Can you work these out from the model? Positions are in its coordinate system, mm. A direction names the side the tool comes from. Round coordinates to 2 decimals unless told otherwise and drop trailing zeros. Order: outer loops, then holes, each group sorted by start corner. A loop starts at its lowest first (then second) coordinate and runs counter-clockwise, first axis right, second up. Notation, with made-up numbers: (-27.5, -16.75) - (-0.5, -16.75) arc R20 ccw to (-0.5, 18.25) - close; hole circle Ø7 at (63.25, 22.25). An arc over 180 degrees is marked (long way). Write item = value, one per line.
Autodesk Fusion 360 part; units mm, degrees
sketch "Sketch1" plane through (0, 0, 0) normal (0, 1, 0) x (1, 0, 0)
  line L0 (0, 0) -> (89, 0)
  line L1 (89, 0) -> (89, -113)
  line L2 (89, -113) -> (0, -113)
  line L3 (0, -113) -> (0, 0)
  line L4 (0, 0) -> (4, 0)
  line L5 (4, 0) -> (4, -4)
  line L6 (4, -4) -> (0, -4)
  line L7 (0, -4) -> (0, 0)
  line L8 (89, 0) -> (85, 0)
  line L9 (85, 0) -> (85, -4)
  line L10 (85, -4) -> (89, -4)
  line L11 (89, -4) -> (89, 0)
  line L12 (89, -113) -> (85, -113)
  line L13 (85, -113) -> (85, -109)
  line L14 (85, -109) -> (89, -109)
  line L15 (89, -109) -> (89, -113)
  line L16 (0, -113) -> (4, -113)
  line L17 (4, -113) -> (4, -109)
  line L18 (4, -109) -> (0, -109)
  line L19 (0, -109) -> (0, -113)
  circle A0 centre (4, -4) radius 1.1
  circle A1 centre (85, -4) radius 1.1
  circle A2 centre (85, -109) radius 1.1
  circle A3 centre (4, -109) radius 1.1
  circle A4 centre (20, -20) radius 2.5
  line L20 (89, 0) -> (69, 0)
  line L21 (69, 0) -> (69, -20)
  line L22 (69, -20) -> (89, -20)
  line L23 (89, -20) -> (89, 0)
  line L24 (0, 0) -> (20, 0)
  line L25 (20, 0) -> (20, -20)
  line L26 (20, -20) -> (0, -20)
  line L27 (0, -20) -> (0, 0)
  line L28 (0, -113) -> (20, -113)
  line L29 (20, -113) -> (20, -93)
  line L30 (20, -93) -> (0, -93)
  line L31 (0, -93) -> (0, -113)
  line L32 (89, -113) -> (69, -113)
  line L33 (69, -113) -> (69, -93)
  line L34 (69, -93) -> (89, -93)
  line L35 (89, -93) -> (89, -113)
  circle A5 centre (69, -20) radius 2.5
  circle A6 centre (20, -93) radius 2.5
  circle A7 centre (69, -93) radius 2.5
  dimension "d1" = 89
  dimension "d2" = 113
  dimension "d3" = 4
  dimension "d4" = 4
  dimension "d5" = 4
  dimension "d6" = 4
  dimension "d7" = 4
  dimension "d8" = 4
  dimension "d9" = 4
  dimension "d10" = 4
  dimension "d11" = 2.2
  dimension "d12" = 2.2
  dimension "d13" = 2.2
  dimension "d14" = 2.2
  dimension "d30" = 5
  dimension "d31" = 20
  dimension "d32" = 20
  dimension "d33" = 20
  dimension "d34" = 20
  dimension "d35" = 20
  dimension "d36" = 20
  dimension "d37" = 5
  dimension "d38" = 5
  dimension "d39" = 5
extrude "Extrude1" add sketch "Sketch1" along normal blind 2
sketch "Sketch2" plane through (0, 2, 0) normal (0, 1, 0) x (-1, 0, 0)
  line L0 (0, 0) -> (0, 113)
  line L1 (0, 113) -> (-89, 113)
  line L2 (-89, 113) -> (-89, 0)
  line L3 (-89, 0) -> (0, 0)
  line L4 (0, 0) -> (-89, 0)
  line L5 (-89, 0) -> (-89, 3.5)
  line L6 (-89, 3.5) -> (0, 3.5)
  line L7 (0, 3.5) -> (0, 0)
  line L8 (0, 0) -> (-3.5, 0)
  line L9 (-3.5, 0) -> (-3.5, 113)
  line L10 (-3.5, 113) -> (0, 113)
  line L11 (0, 113) -> (0, 0)
  line L12 (0, 113) -> (-89, 113)
  line L13 (-89, 113) -> (-89, 109.5)
  line L14 (-89, 109.5) -> (0, 109.5)
  line L15 (0, 109.5) -> (0, 113)
  line L16 (-89, 113) -> (-85.5, 113)
  line L17 (-85.5, 113) -> (-85.5, 0)
  line L18 (-85.5, 0) -> (-89, 0)
  line L19 (-89, 0) -> (-89, 113)
  dimension "d17" = 3.5
  dimension "d18" = 3.5
  dimension "d19" = 3.5
  dimension "d20" = 3.5
extrude "Extrude2" add sketch "Sketch2" along normal blind 33 contours L0 L3 L4 L6 L7 L8 L9 L11 | L0 L6 L9 L11 L14 | L3 L4 L6 L9 L17 | L0 L1 L9 L10 L11 L12 L14 L15 | L2 L3 L4 L5 L6 L17 L18 L19 | L1 L9 L12 L14 L17 | L2 L6 L14 L17 L19 | L1 L2 L12 L13 L14 L16 L17 L19
sketch "Sketch3" plane through (0, 0, 0) normal (-1, 0, 0) x (0, 0, 1)
  line L0 (0, 0) -> (113, 0)
  line L1 (113, 0) -> (113, 35)
  line L2 (113, 35) -> (0, 35)
  line L3 (0, 35) -> (0, 0)
  line L4 (113, 0) -> (113, 9)
  line L5 (113, 9) -> (0, 35)
  dimension "d23" = 9
extrude "Extrude3" cut sketch "Sketch3" against normal blind 92 contours L1 L2 L5
fillet "Fillet1" radius 14 4 edges at (3.5, 18.0973, 3.5) (85.5, 18.0973, 3.5) (85.5, 5.9027, 109.5) (3.5, 5.9027, 109.5)
extrude "Extrude4" cut sketch "Sketch1" along normal blind 50 contours L5 L6 A0 | L5 L6 A0 | L9 L10 A1 | L9 L10 A1 | L17 L18 A3 | L17 L18 A3 | L13 L14 A2 | L13 L14 A2
extrude "Extrude5" cut sketch "Sketch1" along normal blind 5 contours A4 L25 L26 | A4 L25 L26 | L21 L22 A5 | L21 L22 A5 | L29 L30 A6 | L29 L30 A6 | L33 L34 A7 | L33 L34 A7
fillet "Fillet2" radius 3 4 edges at (0, 4.5, 113) (89, 4.5, 113) (89, 17.5, 0) (0, 17.5, 0)
fillet "Fillet3" radius 2 4 edges at (4, 9.6673, 110.1) (85, 9.6673, 110.1) (85, 33.8265, 5.1) (4, 33.8265, 5.1)
sketch "Sketch4" plane through (0, 0, 0) normal (0, 0, -1) x (-1, 0, 0)
  line L0 (-3, 0) -> (-3, 35)
  line L1 (-3, 35) -> (-86, 35)
  line L2 (-86, 35) -> (-86, 0)
  line L3 (-86, 0) -> (-3, 0)
  line L4 (-86, 35) -> (-44.5, 35)
  circle A0 centre (-44.5, 35) radius 4.5
extrude "Extrude6" cut sketch "Sketch4" against normal blind 6 contours L1 L4 A0 picked at (-47.4832, 34.7764)
fillet "Fillet4" radius 1.5 2 edges at (44.5, 30.5, 0) (44.5, 30.5, 3.5)
(1) If I drill on line 1 (Z direction, x = 69, y = 1.25); line 2 (X direction, y = 1.2, z = 20); line 3 (X direction, y = 15, z = 50.5), over which ranges is the centre line in solid material (lowest first)? Write a range as from..to.
Computed:
line_1 = 0..17.5, 22.5..90.5, 95.5..113
line_2 = 0..17.5, 22.5..66.5, 71.5..89
line_3 = 0..3.5, 85.5..89
(2) Thinking about a two-plate mould opening in X: for faces 1 (the face through (7.5, 6.4, 105.3)), 2 (the face through (44, 0, 56)), 3 (the face through (89, 13, 44)), which applies, +X half, -X half, draft (parallel to the pull), parting line (faces both ways), or undercut?
Computed:
face_1 = undercut
face_2 = draft
face_3 = +X half
(3) If we section it at D-D (z = 93): Write out the boundary of the cut face in (x, y), plus the area to 3 significant figures.
Computed:
outline = (0, 0) - (17.5, 0) - (17.5, 2) - (3.5, 2) - (3.5, 13.6) - (0, 13.6) - close; (22.5, 0) - (66.5, 0) - (66.5, 2) - (22.5, 2) - close; (71.5, 0) - (89, 0) - (89, 13.6) - (85.5, 13.6) - (85.5, 2) - (71.5, 2) - close
area = 239 mm^2
(4) Will these pins go through, and if not, where does the flat tip stop? P1, Ø4.5, axis at x = 69, z = 93, coming from the +Y side; P2, Ø8, axis at y = 20.5, z = 60, coming from the -X side; P3, Ø6, axis at x = 20, y = 24.5, coming from the +Z side; P4, Ø6.5, axis at x = 69, z = 20, coming from the +Y side.
Computed:
P1 = through
P2 = 0
P3 = 3.51
P4 = 2
(5) If we section it at C-C (x = 37): Write out the boundary of the cut face in (y, z), plus the area to 3 significant figures.
Computed:
outline = (0, 0) - (35, 0) - (34.19, 3.5) - (2, 3.5) - (2, 109.5) - (9.81, 109.5) - (9, 113) - (0, 113) - close
area = 366 mm^2
(6) If we section it at B-B (y = 17.5): Write out the boundary of the cut face in (x, z).
Computed:
outline = (0, 3) arc R3 ccw to (3, 0) - (86, 0) arc R3 ccw to (89, 3) - (89, 76.06) - (85.5, 76.06) - (85.5, 17.5) arc R14 cw to (71.5, 3.5) - (17.5, 3.5) arc R14 cw to (3.5, 17.5) - (3.5, 76.06) - (0, 76.06) - close; hole circle Ø2.2 at (4, 4); hole circle Ø2.2 at (85, 4)
(7) On a 3-axis mill with a long thin cutter (end or side, diameter ignored), from which of +Z, -Z, +X, -X, +Y, -Y can I reach the whole of each face in a straight line? I mean faces 4 (the face through (81.5, 18.3, 7.7)), 5 (the face through (19.67, 0.99, 95.48)). Say none if no direction works.
Computed:
face_4 = +Y
face_5 = +Y, -Y
(8) If we section it at A-A (x = 20): Write out the boundary of the cut face in (y, z).
Computed:
outline = (0, 0) - (35, 0) - (34.19, 3.5) - (2, 3.5) - (2, 17.5) - (0, 17.5) - close; (0, 22.5) - (2, 22.5) - (2, 90.5) - (0, 90.5) - close; (0, 95.5) - (2, 95.5) - (2, 109.5) - (9.81, 109.5) - (9, 113) - (0, 113) - close
